Autodesk Inventor part; units mm, degrees
ref_plane "YZ Plane" through (0, 0, 0) normal (1, 0, 0) x (0, 1, 0)
ref_plane "XZ Plane" through (0, 0, 0) normal (0, 1, 0) x (-1, 0, 0)
ref_plane "XY Plane" through (0, 0, 0) normal (0, 0, 1) x (1, 0, 0)
sketch "Boceto1" plane through (0, 0, 0) normal (0, 0, 1) x (1, 0, 0)
  line L0 (0, 5) -> (0, 145)
  line L1 (5, 150) -> (30, 150)
  line L2 (35, 145) -> (35, 5)
  line L3 (30, 0) -> (5, 0)
  arc A0 (5, 150) -> (0, 145) centre (5, 145) ccw
  arc A1 (35, 145) -> (30, 150) centre (30, 145) ccw
  arc A2 (0, 5) -> (5, 0) centre (5, 5) ccw
  arc A3 (30, 0) -> (35, 5) centre (30, 5) ccw
  circle A4 centre (17.5, 120) radius 4.5
  circle A5 centre (17.5, 100) radius 2.5
  circle A6 centre (17.5, 80) radius 2.5
  circle A7 centre (17.5, 20) radius 6.5
  circle A8 centre (22.5, 54.5) radius 2.5
  circle A9 centre (12.5, 54.5) radius 2.5
  circle A10 centre (12.5, 6) radius 2.5
  circle A11 centre (22.5, 6) radius 2.5
  circle A12 centre (6, 127) radius 1.25
  circle A13 centre (6, 113) radius 1.25
  circle A14 centre (29, 113) radius 1.25
  circle A15 centre (29, 127) radius 1.25
  point P0 (0, 0)
extrude "Extrusión1" add sketch "Boceto1" along normal blind 3
sketch "Boceto2" plane through (0, 0, 0) normal (0, 0, -1) x (-1, 0, 0)
  circle A0 centre (-17.5, 20) radius 6.5
  arc A1 (-27, 23.1225) -> (-8, 23.1225) centre (-17.5, 20) ccw
  line L0 (-17.5, 47) -> (-27, 47)
  line L1 (-27, 47) -> (-8, 47)
  line L2 (-8, 47) -> (-8, 23.1225)
  line L3 (-27, 47) -> (-27, 23.1225)
  point P0 (0, 0)
extrude "Extrusión2" cut sketch "Boceto2" against normal blind 10
properties part number "3"
Geometry: final body of the model. Coordinates: model frame, mm. A direction names the side the tool comes from. Round coordinates to 2 decimals unless told otherwise and drop trailing zeros. Order: outer loops, then holes, each group sorted by start corner. A loop starts at its lowest first (then second) coordinate and runs counter-clockwise, first axis right, second up.
Q1. Access query for faces 1 (the face through (27, 35, 1)), 2 (the face through (18, 0, 1)). Directions: +Z, -Z, +X, -X, +Y, -Y. A direction counts if a zero-diameter tool reaches every point of the face in a straight line with its end or side. Return the directions, or none.
Result sheet:
face 1: +Z, -Z
face 2: +Z, -Z, +X, -X, -Y
Q2. Section C-C, the plane z = 1.6. Give the number of separate pieces and of enclosed holes in the cut face, and give its area (3 significant figures).
Result sheet:
separate pieces: 1
enclosed holes: 12
area: 4,360 mm2
Q3. Section D-D, the plane x = 16.5. Output: boundary loops of the cut face in (y, z), and give its area (3 significant figures).
Result sheet:
outline: (0, 0) - (10.05, 0) - (10.05, 3) - (0, 3) - close; (47, 0) - (77.71, 0) - (77.71, 3) - (47, 3) - close; (82.29, 0) - (97.71, 0) - (97.71, 3) - (82.29, 3) - close; (102.29, 0) - (115.61, 0) - (115.61, 3) - (102.29, 3) - close; (124.39, 0) - (150, 0) - (150, 3) - (124.39, 3) - close
area: 285 mm2
Q4. Section B-B, the plane y = 30. Output: boundary loops of the cut face in (x, z).
Result sheet:
outline: (0, 0) - (8, 0) - (8, 3) - (0, 3) - close; (27, 0) - (35, 0) - (35, 3) - (27, 3) - close
Q5. Mould query, pull axis X, two halves, no side actions, for faces 3 (the face through (15, 80, 1)), 4 (the face through (17, 76, 0)), 5 (the face through (1, 148, 1)), 6 (the face through (17.17, 97.52, 1.48)). Classes: released by +X, released by -X, zero draft, split by the parting line, or undercut.
Result sheet:
face 3: undercut
face 4: zero draft
face 5: released by -X
face 6: undercut
Q6. Section A-A, the plane y = 127. Output: boundary loops of the cut face in (x, z).
Result sheet:
outline: (0, 0) - (4.75, 0) - (4.75, 3) - (0, 3) - close; (7.25, 0) - (27.75, 0) - (27.75, 3) - (7.25, 3) - close; (30.25, 0) - (35, 0) - (35, 3) - (30.25, 3) - close
Q7. Material intervals for probe 1 along X at (y, z) = (127, 1.5); probe 2 along Y at (x, z) = (17.5, 0.6); probe 3 along Y at (x, z) = (13.5, 0.9), sorted ascending.
Result sheet:
probe 1: x = 0 to 4.75, 7.25 to 27.75, 30.25 to 35
probe 2: y = 0 to 10, 47 to 77.5, 82.5 to 97.5, 102.5 to 115.5, 124.5 to 150
probe 3: y = 0 to 3.71, 8.29 to 10.83, 47 to 52.21, 56.79 to 117.94, 122.06 to 150
